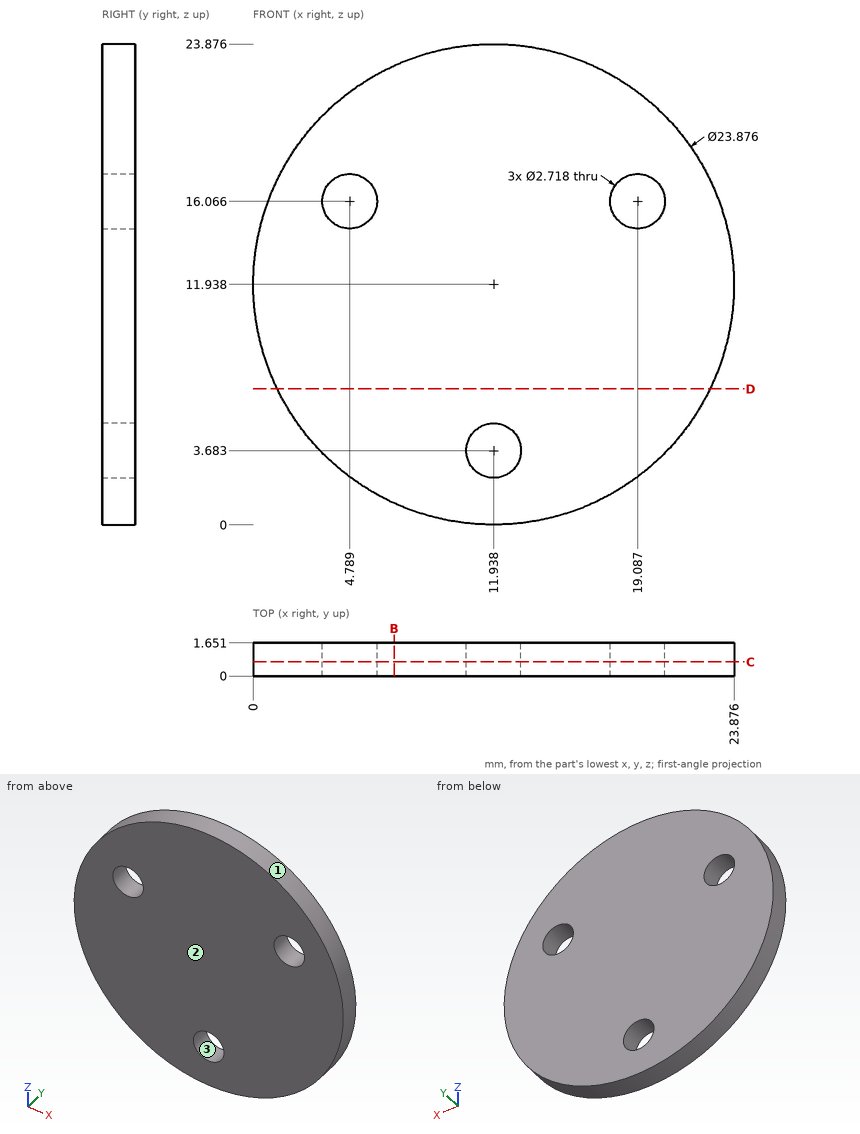
The figure shows three views and two pictorial views of one solid part (mm, origin at its lowest corner). Answer the questions. Round coordinates to 2 decimals unless told otherwise and drop trailing zeros. Order: outer loops, then holes, each group sorted by start corner. A loop starts at its lowest first (then second) coordinate and runs counter-clockwise, first axis right, second up. Notation, with made-up numbers: M 21,-4.5 L 77,-4.5 A22 ccw 77,5.5 Z; hole C -33.5,-12.75 d3. An arc over 180 degrees is marked long. Put each result on its own line as item: value. Start each with the question number.
Q1. Straight lines are drawn through the part: L1, parallel to X at y = 0.8, z = 16 (1 decimal); L2, parallel to X at y = 0.75, z = 12 (1 decimal); L3, parallel to Z at x = 11.5, y = 0.15 (1 decimal). For each, find the intervals that lie inside material, in ascending order. Write a range as [from, to].
Q2. A flat-ended cylindrical pin translates along its axis: pin 1 (1.6 mm diameter, centred on x = 4.79, z = 16.07, fed in from -Y). Find the tip coordinate at first contact, or state that the pin passes through.
Q3. Section C-C, the plane y = 0.7 is taken. Write down the section's boundary in (x, z) (1 decimal).
Q4. For a pull along Z with two mould halves and no side action, classify the marked faces 1, 2 and 3 as pulls with the +Z half, pulls with the -Z half, needs draft (parallel to the pull), parting line crosses it, or undercut.
Q5. Section B-B, the plane x = 7 is taken. Write down the section's boundary in (y, z).
Q6. Section D-D, the plane z = 6.75 is taken. Write down the section's boundary in (x, y).
Findings below:
1. L1: x = [0.7, 3.4], [6.1, 17.7], [20.4, 23.2]
1. L2: x = [0, 23.9]
1. L3: z = [0, 2.4], [5, 23.9]
2. pin 1: passes through
3. outline: C 11.9,11.9 d23.9; hole C 4.8,16.1 d2.7; hole C 11.9,3.7 d2.7; hole C 19.1,16.1 d2.7
4. face 1: parting line crosses it
4. face 2: needs draft
4. face 3: undercut
5. outline: M 0,1.07 L 1.65,1.07 L 1.65,22.81 L 0,22.81 Z
6. outline: M 1.19,0 L 22.69,0 L 22.69,1.65 L 1.19,1.65 Z
